Work out the finished part from the listing and answer in its coordinate system (mm). Round coordinates to 2 decimals unless told otherwise and drop trailing zeros. Write each loop counter-clockwise with the first axis right and the second up, starting at its lowest first coordinate (ties: lowest second). Pieces come first, ordered by that corner, then holes.
1. Find section C-C (x = 27.5). Write down the section's boundary in (y, z).
2. Flat-ended cylindrical pins translate along their axes: pin 1 Ø1.5 at (x, z) = (-29, 6) entering from -Y; pin 2 Ø1.5 at (y, z) = (-5.5, 5) entering from -X; pin 3 Ø1.8 at (y, z) = (-5, 4.5) entering from +X. Find the tip coordinate at first contact, or state that the pin passes through.
3. Straight lines are drawn through the part: probe 1 along Y at (x, z) = (-28, 2.5); probe 2 along Y at (x, z) = (22, 3); probe 3 along Z at (x, y) = (-19.5, 6). For each, find the intervals that lie inside material, in ascending order.
4. Find section B-B (z = 2.25). Count the separate pieces of the cut face and the enclosed holes in it, and give its area (3 significant figures).
5. Find section A-A (x = 12.5). Write down the section's boundary in (y, z).
6. Find section D-D (y = -9.75). Write down the section's boundary in (x, z).
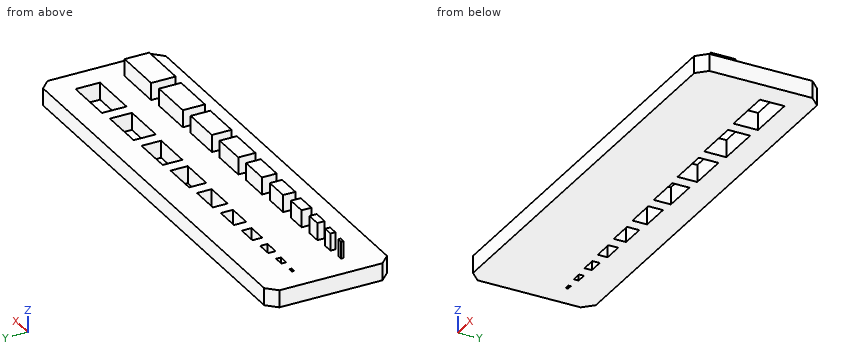
```python
from build123d import *

# Parameters (mm, degrees)
F0_W     = 87.5
F0_H     = 25
F0_W_2   = 1
F0_H_2   = 0.5
F0_W_3   = 2
F0_H_3   = 1
F0_W_4   = 3
F0_H_4   = 1.5
F0_W_5   = 4
F0_H_5   = 2
F0_W_6   = 5
F0_H_6   = 2.5
F0_W_7   = 6
F0_H_7   = 3
F0_W_8   = 7
F0_H_8   = 3.5
F0_W_9   = 8
F0_H_9   = 4
F0_W_10  = 9
F0_H_10  = 4.5
F0_W_11  = 10
F0_H_11  = 5
F1_DEPTH = 3.5
F2_DEPTH = 7
F3_SIZE  = 2


with BuildPart() as f1:
    # F0 (on Top) → F1 (new body)
    with BuildSketch(Plane.XY):
        Rectangle(F0_W, F0_H)
        with Locations((-38.25, -5)):
            Rectangle(F0_W_2, F0_H_2, mode=Mode.SUBTRACT)
        with Locations((-34.25, -5)):
            Rectangle(F0_W_3, F0_H_3, mode=Mode.SUBTRACT)
        with Locations((-29.25, -5)):
            Rectangle(F0_W_4, F0_H_4, mode=Mode.SUBTRACT)
        with Locations((-23.25, -5)):
            Rectangle(F0_W_5, F0_H_5, mode=Mode.SUBTRACT)
        with Locations((-16.25, -5)):
            Rectangle(F0_W_6, F0_H_6, mode=Mode.SUBTRACT)
        with Locations((-8.25, -5)):
            Rectangle(F0_W_7, F0_H_7, mode=Mode.SUBTRACT)
        with Locations((0.75, -5)):
            Rectangle(F0_W_8, F0_H_8, mode=Mode.SUBTRACT)
        with Locations((10.75, -5)):
            Rectangle(F0_W_9, F0_H_9, mode=Mode.SUBTRACT)
        with Locations((21.75, -5)):
            Rectangle(F0_W_10, F0_H_10, mode=Mode.SUBTRACT)
        with Locations((33.75, -5)):
            Rectangle(F0_W_11, F0_H_11, mode=Mode.SUBTRACT)
        Polygon((-38.25, 5.25), (-37.75, 5.25), (-37.75, 4.75), (-38.75, 4.75), (-38.75, 5.25), align=None, mode=Mode.SUBTRACT)
        Polygon((-34.25, 5.5), (-33.25, 5.5), (-33.25, 4.5), (-35.25, 4.5), (-35.25, 5.5), align=None, mode=Mode.SUBTRACT)
        Polygon((-30.75, 4.25), (-30.75, 5.75), (-29.25, 5.75), (-27.75, 5.75), (-27.75, 4.25), align=None, mode=Mode.SUBTRACT)
        Polygon((-25.25, 4), (-25.25, 6), (-23.25, 6), (-21.25, 6), (-21.25, 4), align=None, mode=Mode.SUBTRACT)
        Polygon((-18.75, 3.75), (-18.75, 6.25), (-16.25, 6.25), (-13.75, 6.25), (-13.75, 3.75), align=None, mode=Mode.SUBTRACT)
        Polygon((-11.25, 3.5), (-11.25, 6.5), (-8.25, 6.5), (-5.25, 6.5), (-5.25, 3.5), align=None, mode=Mode.SUBTRACT)
        Polygon((-2.75, 3.25), (-2.75, 6.75), (0.75, 6.75), (4.25, 6.75), (4.25, 3.25), align=None, mode=Mode.SUBTRACT)
        Polygon((6.75, 3), (6.75, 7), (10.75, 7), (14.75, 7), (14.75, 3), align=None, mode=Mode.SUBTRACT)
        Polygon((17.25, 2.75), (17.25, 7.25), (21.75, 7.25), (26.25, 7.25), (26.25, 2.75), align=None, mode=Mode.SUBTRACT)
        Polygon((28.75, 2.5), (28.75, 7.5), (33.75, 7.5), (38.75, 7.5), (38.75, 2.5), align=None, mode=Mode.SUBTRACT)
    extrude(amount=F1_DEPTH)

    # F0 (on Top) → F2 (join, through all)
    with BuildSketch(Plane.XY):
        with Locations((-38.25, -5)):
            Rectangle(F0_W_2, F0_H_2)
        with Locations((-34.25, -5)):
            Rectangle(F0_W_3, F0_H_3)
        with Locations((-29.25, -5)):
            Rectangle(F0_W_4, F0_H_4)
        with Locations((-23.25, -5)):
            Rectangle(F0_W_5, F0_H_5)
        with Locations((-16.25, -5)):
            Rectangle(F0_W_6, F0_H_6)
        with Locations((-8.25, -5)):
            Rectangle(F0_W_7, F0_H_7)
        with Locations((0.75, -5)):
            Rectangle(F0_W_8, F0_H_8)
        with Locations((10.75, -5)):
            Rectangle(F0_W_9, F0_H_9)
        with Locations((21.75, -5)):
            Rectangle(F0_W_10, F0_H_10)
        with Locations((33.75, -5)):
            Rectangle(F0_W_11, F0_H_11)
    extrude(amount=F2_DEPTH)

    # F3
    f3_edges = [f1.edges().sort_by_distance(p)[0] for p in [
        (-43.75, -12.5, 1.75),
        (43.75, -12.5, 1.75),
        (43.75, 12.5, 1.75),
        (-43.75, 12.5, 1.75),
    ]]
    chamfer(f3_edges, length=F3_SIZE)


solid = f1.part
```
Worked answers:
1. outline: (-12.5, 0) - (12.5, 0) - (12.5, 3.5) - (-12.5, 3.5) - close
2. pin 1: stops at y = -5.75
2. pin 2: stops at x = -38.75
2. pin 3: stops at x = 38.75
3. probe 1: y = -12.5 to 4.25, 5.75 to 12.5
3. probe 2: y = -12.5 to 2.75, 7.25 to 12.5
3. probe 3: z = 0 to 3.5
4. separate pieces: 1
4. enclosed holes: 10
4. area: 1,990 mm2
5. outline: (-12.5, 0) - (3, 0) - (3, 3.5) - (-3, 3.5) - (-3, 7) - (-7, 7) - (-7, 3.5) - (-12.5, 3.5) - close; (7, 0) - (12.5, 0) - (12.5, 3.5) - (7, 3.5) - close
6. outline: (-43.75, 0) - (43.75, 0) - (43.75, 3.5) - (-43.75, 3.5) - close
